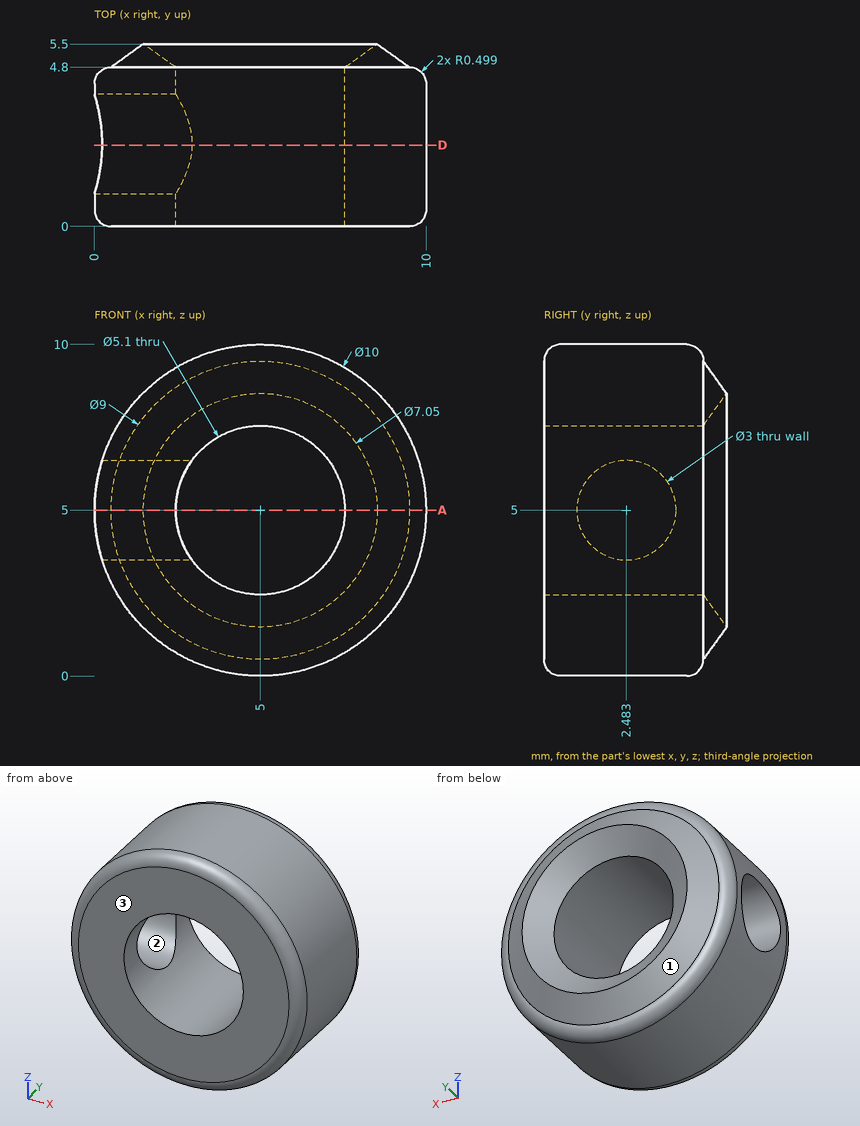
Study the drawing (mm; zero at the part's minimum x, y, z) and answer. Give positions to 0.01 mm unless a question says otherwise; leave off trailing zeros. Order: outer loops, then holes, each group sorted by start corner. A loop starts at its lowest first (then second) coordinate and runs counter-clockwise, first axis right, second up. Notation, with made-up numbers: (-14, 45) - (24, 45) arc R34 ccw to (24, 84) - close; hole circle Ø5 at (-5, 14.25). An arc over 180 degrees is marked (long way). Use one line per item in the form item = value. Start each with the question number.
(1) A flat-ended cylindrical pin translates along its axis: pin 1 Ø2 at (x, z) = (7, 4) entering from +Y. Find the tip coordinate at first contact, or state that the pin passes through.
(2) A cutting plane is placed at D-D, the plane y = 2.45. Write down the section's boundary in (x, z).
(3) The mould has two halves that part along Y. Classify the marked faces 1, 2 and 3: released by +Y, released by -Y, zero draft, split by the parting line, or undercut.
(4) Consider line 1 (Z direction, x = 5, y = 1.4); line 2 (Z direction, x = 6.5, y = 4.55); line 3 (X direction, y = 0.75, z = 3.5). Determine where each line is inside the solid, lowest interval first. Write a range as from..to.
(5) A cutting plane is placed at A-A, the plane z = 5. State how many separate pieces and enclosed holes the cut face has, then the cut area to 3 significant figures.
Ans:
q1.pin_1 = 5.29
q2.outline = (0.23, 3.5) arc R5 ccw (long way) to (0.23, 6.5) - (2.94, 6.5) arc R2.55 cw (long way) to (2.94, 3.5) - close
q3.face_1 = released by +Y
q3.face_2 = undercut
q3.face_3 = released by -Y
q4.line_1 = 0..2.45, 7.55..10
q4.line_2 = 0.3..2.94, 7.06..9.7
q4.line_3 = 0.23..2.94, 7.06..9.77
q5.separate_pieces = 3
q5.enclosed_holes = 0
q5.area = 17.3 mm^2
